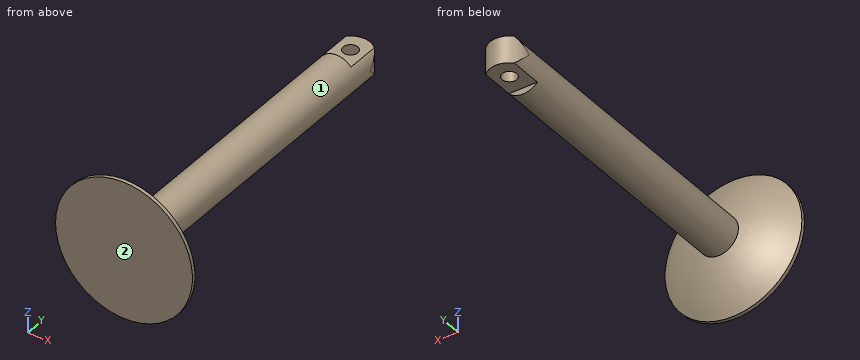
```python
from build123d import *

# Parameters (mm, degrees)
SKETCH1_W               = 4
SKETCH1_H               = 65
CUT_EXTRUDE2_DEPTH      = 15.0000001
CUT_EXTRUDE2_DEPTH_BACK = 15.0000001
SKETCH3_W               = 1.25
SKETCH3_H               = 8
CUT_EXTRUDE3_DEPTH      = 15.0000001
CUT_EXTRUDE3_DEPTH_BACK = 15.0000001


with BuildPart() as part:
    # Sketch1 → Revolve1 (revolve)
    with BuildSketch(Plane.XY):
        with BuildLine():
            ThreePointArc((-4, -65), (-9.225090437, -66.601484736), (-14, -69.259785338))
            Line((-14, -69.259785338), (-14, -70))
            Line((-14, -70), (0, -70))
            Line((0, -70), (0, -65))
            Line((0, -65), (-4, -65))
        make_face()
        with Locations((-2, -32.5)):
            Rectangle(SKETCH1_W, SKETCH1_H)
    revolve(axis=Axis((0, 0, 0), (0, -1, 0)))

    # Sketch2 → Cut-Extrude2 (cut, two sides)
    with BuildSketch(Plane.XY) as cut_extrude2_sk:
        with BuildLine():
            Line((-4, 0), (-4, -4))
            ThreePointArc((-4, -4), (-2.828427125, -1.171572875), (0, 0))
            Line((0, 0), (-4, 0))
        make_face()
        with BuildLine():
            ThreePointArc((0, 0), (2.828427125, -1.171572875), (4, -4))
            Line((4, -4), (4, 0))
            Line((4, 0), (0, 0))
        make_face()
        with BuildLine():
            ThreePointArc((-1.5, -4), (0, -5.5), (1.5, -4))
            Line((1.5, -4), (-1.5, -4))
        make_face()
        with BuildLine():
            Line((-1.5, -4), (1.5, -4))
            ThreePointArc((1.5, -4), (0, -2.5), (-1.5, -4))
        make_face()
    extrude(amount=CUT_EXTRUDE2_DEPTH, mode=Mode.SUBTRACT)
    extrude(cut_extrude2_sk.sketch, amount=-CUT_EXTRUDE2_DEPTH_BACK, mode=Mode.SUBTRACT)

    # Sketch3 → Cut-Extrude3 (cut, two sides)
    with BuildSketch(Plane(origin=(0, 0, 0), x_dir=(0, 0, -1), z_dir=(1, 0, 0))) as cut_extrude3_sk:
        with Locations((-3.375, -4)):
            Rectangle(SKETCH3_W, SKETCH3_H)
        with Locations((3.375, -4)):
            Rectangle(SKETCH3_W, SKETCH3_H)
    extrude(amount=CUT_EXTRUDE3_DEPTH, mode=Mode.SUBTRACT)
    extrude(cut_extrude3_sk.sketch, amount=-CUT_EXTRUDE3_DEPTH_BACK, mode=Mode.SUBTRACT)


solid = part.part
```
Source: CAD feature listing. Evaluate the final solid. Frame: model axes, mm. Face numbers are marked on the shaded views. A direction names the side the tool comes from. Coordinates: 2 decimals unless noted, no trailing zeros. Loops run counter-clockwise (first coordinate to the right, second up) from the corner with the lowest first, then second, coordinate; pieces in that order, holes last. Notation, with made-up numbers: M 9.5,40.5 L 42.5,40.5 A18 ccw 42.5,45.5 Z; hole C 56.5,76.25 d4. An arc over 180 degrees is marked long. Put each result on its own line as item: value. Start each with the question number.
1) Ray query, L1, parallel to Y at x = 0, z = 0.2; L2, parallel to X at y = -4, z = 0; L3, parallel to X at y = -4, z = -0.7. Return the intervals inside material, ascending. Write a range as from..to.
2) Contact query for flat-ended pins moving along their axis: pin 1 Ø1.4 at (x, z) = (-1, 3) entering from +Y (3 decimals); pin 2 Ø6.5 at (x, y) = (1, -5) entering from +Z; pin 3 Ø1 at (y, z) = (-51, 0.5) entering from -X. Output: stop coordinate, or through.
3) Reachability of the marked faces 1 and 2 from +Z, -Z, +X, -X, +Y, -Y: full face, straight path, thin tool, end or side. Return the list, or none.
4) Cut plane A-A on y = -42. Return the cut outline in (x, z), then the cut area to 3 significant figures.
The answers:
1. L1: y = -70..-5.5, -2.5..0
1. L2: x = -4..-1.5, 1.5..4
1. L3: x = -3.94..-1.5, 1.5..3.94
2. pin 1: stops at y = -0.015
2. pin 2: stops at z = 4
2. pin 3: stops at x = -4
3. face 1: +Y
3. face 2: +Z, -Z, +X, -X, -Y
4. outline: C 0,0 d8
4. area: 50.3 mm²
